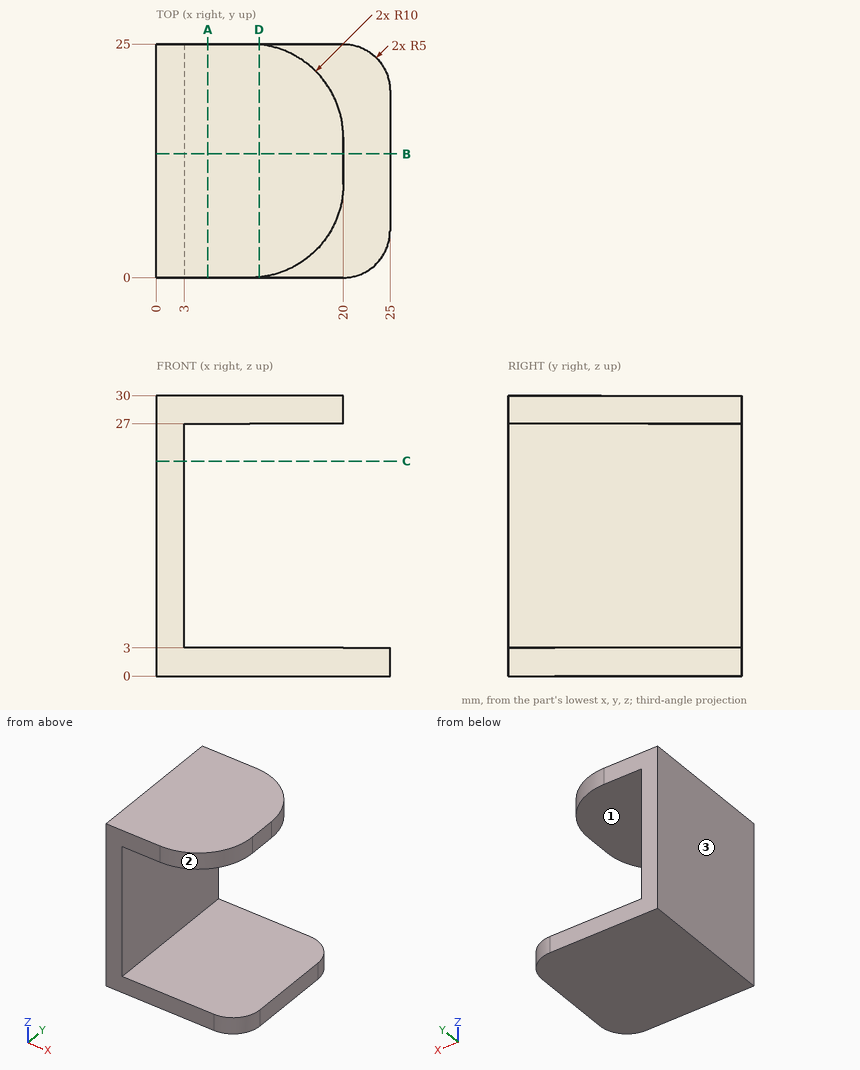
Check sheet for the drawn part. Datum: minimum x, y, z corner. Units: mm. A direction names the side the tool comes from. Round coordinates to 2 decimals unless told otherwise and drop trailing zeros. Loops run counter-clockwise (first coordinate to the right, second up) from the corner with the lowest first, then second, coordinate; pieces in that order, holes last.
Item 1: Cross-section at B-B on y = 13.25. Record the boundary of the cut face in (x, z).
Item 2: Cross-section at C-C on z = 23. Record the boundary of the cut face in (x, y).
Item 3: Access from +Z, -Z, +X, -X, +Y, -Y to the whole of each face (thin tool, end or side, straight path). Record for the marked faces 1, 2 and 3.
Item 4: Cross-section at D-D on x = 11. Record the boundary of the cut face in (y, z).
Item 5: Gauge pin test, flat ends, axial feed: pin 1 (4 mm diameter, centred on y = 17.5, z = 13, fed in from +X); pin 2 (2.5 mm diameter, centred on y = 13.5, z = 28, fed in from +X). Record the tip position at first contact, or that the pin passes through.
Item 6: Thickness scan on line 1 (Z direction, x = 6, y = 6.75); line 2 (X direction, y = 16.5, z = 20.25). Record the ranges inside material, lowest first.
Item 7: Cross-section at A-A on x = 5.5. Record the boundary of the cut face in (y, z).
Answer sheet:
1. outline: (0, 0) - (25, 0) - (25, 3) - (3, 3) - (3, 27) - (20, 27) - (20, 30) - (0, 30) - close
2. outline: (0, 0) - (3, 0) - (3, 25) - (0, 25) - close
3. face 1: +X, +Y, -Y
3. face 2: +Z, +X, -Y
3. face 3: +Z, -Z, -X, +Y, -Y
4. outline: (0, 0) - (25, 0) - (25, 3) - (0, 3) - close; (0.05, 27) - (24.95, 27) - (24.95, 30) - (0.05, 30) - close
5. pin 1: stops at x = 3
5. pin 2: stops at x = 20
6. line 1: z = 0 to 3, 27 to 30
6. line 2: x = 0 to 3
7. outline: (0, 0) - (25, 0) - (25, 3) - (0, 3) - close; (0, 27) - (25, 27) - (25, 30) - (0, 30) - close
